Part model, mm, in its own coordinate system. Face numbers are marked on the shaded views. A direction names the side the tool comes from. Round coordinates to 2 decimals unless told otherwise and drop trailing zeros. Loops run counter-clockwise (first coordinate to the right, second up) from the corner with the lowest first, then second, coordinate; pieces in that order, holes last.
(1) Probe probe 1 along X at (y, z) = (15.5, -262.25); probe 2 along Y at (x, z) = (-152, -259); probe 3 along Y at (x, z) = (-153.5, -254.75). List the from-to ranges inside material, lowest first.
(2) Tool access for the marked faces 1 and 2: list every direction of +Z, -Z, +X, -X, +Y, -Y with a clear straight run to the whole face (end or side of a thin tool).
(3) Cut at A-A on y = 9. List the corners of the cut face in (x, z), then the cut area to 3 significant figures.
(4) Flat gauge pins, fed straight in: pin 1 (1 mm diameter, centred on x = -150.5, y = 16.5, fed in from -Z); pin 2 (8 mm diameter, centred on x = -158, y = 18.5, fed in from -Z); pin 3 (6 mm diameter, centred on x = -141.5, y = 14.5, fed in from -Z). Where does each tip first touch, or does it go through?
(5) Cut at B-B on y = 21.5. List the corners of the cut face in (x, z), then the cut area to 3 significant figures.
Autodesk Inventor part; units mm, degrees
ref_plane "YZ Plane" through (0, 0, 0) normal (1, 0, 0) x (0, 1, 0)
ref_plane "XZ Plane" through (0, 0, 0) normal (0, 1, 0) x (-1, 0, 0)
ref_plane "XY Plane" through (0, 0, 0) normal (0, 0, 1) x (1, 0, 0)
ref_plane "Work Plane1" through (-149.1228, -3.9521, -261.8445) normal (0, 1, 0) x (1, 0, 0)
sketch "Sketch1" plane through (-149.1228, -3.9521, -261.8445) normal (0, 1, 0) x (1, 0, 0)
  circle A0 centre (0, 0) radius 11
  point P0 (149.1228, -261.8445)
  dimension "d0" = 22
extrude "Extrusion1" add sketch "Sketch1" along normal blind 32
sketch "Sketch2" plane through (-149.1228, 28.0479, -261.8445) normal (0, 1, 0) x (1, 0, 0)
  circle A0 centre (0, 0) radius 1
  point P0 (149.1228, -261.8445)
  dimension "d3" = 2
extrude "Extrusion2" [suppressed]
sketch "Sketch3" plane through (-149.1228, -3.9521, -261.8445) normal (0, -1, 0) x (1, 0, 0)
  circle A0 centre (0, 0) radius 11
  circle A1 centre (0, 0) radius 10.25
  point P0 (149.1228, 261.8445)
  dimension "d6" = 22
  dimension "d7" = 20.5
extrude "Extrusion3" cut sketch "Sketch3" against normal blind 6
chamfer "Chamfer1" distance 8 angle 45 1 edges at (-160.1228, 28.0479, -261.8445)
sketch "Sketch4" plane through (-149.1228, 28.0479, -261.8445) normal (0, 1, 0) x (1, 0, 0)
  circle A0 centre (0, 0) radius 11
  circle A1 centre (0, 0) radius 1.5
  point P0 (149.1228, -261.8445)
  dimension "d13" = 3
extrude "Extrusion4" cut sketch "Sketch4" against normal blind 1 contours A1
fillet "Fillet1" radius 1 1 edges at (-150.6228, 27.0479, -261.8445)
properties part number "Objective_placeholder_V2"
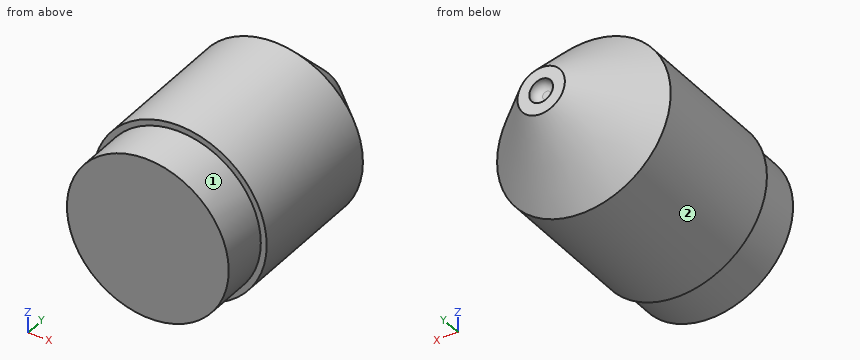
Final values:
1. probe 1: x = -160.12 to -138.13
1. probe 2: y = -3.95 to 27
1. probe 3: y = -3.95 to 22.71
2. face 1: -Y
2. face 2: +Y, -Y
3. outline: circle Ø22 at (-149.12, -261.84)
3. area: 380 mm2
4. pin 1: stops at z = -272.81
4. pin 2: stops at z = -271.7
4. pin 3: stops at z = -271.83
5. outline: circle Ø19.1 at (-149.12, -261.84)
5. area: 286 mm2
